The model under review builds one solid part; all positions refer to its coordinate system, in mm. Face numbers are marked on the shaded views. A direction names the side the tool comes from. Give positions to 0.01 mm unless a question says otherwise; leave off trailing zeros. Order: outer loops, then holes, each group sorted by start corner. A loop starts at its lowest first (then second) coordinate and runs counter-clockwise, first axis right, second up.
```python
from build123d import *

# Parameters (mm, degrees)
SKETCH1_W           = 16
SKETCH1_H           = 20
BOSS_EXTRUDE1_DEPTH = 15
SHELL1_T            = -2
SKETCH10_W          = 2
SKETCH10_H          = 16
BOSS_EXTRUDE4_DEPTH = 14
CUT_EXTRUDE2_REACH  = 32.726
SKETCH3_W           = 15
SKETCH3_H           = 6
CHAMFER1_SIZE       = 1
SKETCH4_W           = 4
SKETCH4_H           = 4
SKETCH4_W_2         = 22
SKETCH4_H_2         = 1.5
BOSS_EXTRUDE2_DEPTH = 2
CUT_EXTRUDE3_REACH  = 28.249
SKETCH5_W           = 12
SKETCH5_H           = 11.5
SKETCH8_R           = 1.75
CUT_EXTRUDE5_DEPTH  = 33.619012861
SKETCH9_R           = 3.25
CUT_EXTRUDE6_DEPTH  = 2.5


with BuildPart() as part:
    # Sketch1 → Boss-Extrude1 (new, symmetric)
    with BuildSketch(Plane.XY):
        Rectangle(SKETCH1_W, SKETCH1_H)
    extrude(amount=BOSS_EXTRUDE1_DEPTH, both=True)

    # Shell1
    shell1_openings = [part.faces().sort_by_distance(p)[0] for p in [
        (-8, 0, 0),
    ]]
    offset(amount=SHELL1_T, openings=shell1_openings, kind=Kind.INTERSECTION)

    # Sketch10 → Boss-Extrude4 (add)
    with BuildSketch(Plane.ZY.offset(-6)):
        with Locations((-12, 0)):
            Rectangle(SKETCH10_W, SKETCH10_H)
        with Locations((12, 0)):
            Rectangle(SKETCH10_W, SKETCH10_H)
    extrude(amount=BOSS_EXTRUDE4_DEPTH)

    # Sketch3 → Cut-Extrude2 (cut, up to next)
    with BuildSketch(Plane(origin=(8, 0, 9.25), x_dir=(0, 0, 1), z_dir=(-1, 0, 0)), mode=Mode.PRIVATE) as cut_extrude2_sk1:
        with Locations((-11.25, 1)):
            Rectangle(SKETCH3_W, SKETCH3_H)
    cut_extrude2_tool1 = extrude(cut_extrude2_sk1.sketch, amount=CUT_EXTRUDE2_REACH, mode=Mode.PRIVATE) & part.part
    add(cut_extrude2_tool1.solids().sort_by_distance((8, 1, -2))[0], mode=Mode.SUBTRACT)

    # Chamfer1
    chamfer1_edges = [part.edges().sort_by_distance(p)[0] for p in [
        (0, -10, 15),
        (8, 0, 15),
        (0, -10, -15),
        (0, 10, -15),
        (8, 0, -15),
        (0, 10, 15),
        (8, -10, 0),
        (8, 10, 0),
    ]]
    chamfer(chamfer1_edges, length=CHAMFER1_SIZE)

    # Sketch4 → Boss-Extrude2 (add)
    with BuildSketch(Plane.ZY.offset(-6)):
        with Locations((-9, 6)):
            Rectangle(SKETCH4_W, SKETCH4_H)
        with Locations((9, 6)):
            Rectangle(SKETCH4_W, SKETCH4_H)
        with Locations((0, -2.75)):
            Rectangle(SKETCH4_W_2, SKETCH4_H_2)
    extrude(amount=BOSS_EXTRUDE2_DEPTH)

    # Sketch5 → Cut-Extrude3 (cut, up to next)
    with BuildSketch(Plane.XZ.offset(10), mode=Mode.PRIVATE) as cut_extrude3_sk1:
        with Locations((-2, 5.25)):
            Rectangle(SKETCH5_W, SKETCH5_H)
    cut_extrude3_tool1 = extrude(cut_extrude3_sk1.sketch, amount=-CUT_EXTRUDE3_REACH, mode=Mode.PRIVATE) & part.part
    add(cut_extrude3_tool1.solids().sort_by_distance((-2, -10, 5.25))[0], mode=Mode.SUBTRACT)

    # Sketch8 → Cut-Extrude5 (cut, through all)
    with BuildSketch(Plane(origin=(0, 0, -15), x_dir=(-1, 0, 0), z_dir=(0, 0, -1))):
        with Locations((3.5, 0)):
            Circle(SKETCH8_R)
    extrude(amount=-CUT_EXTRUDE5_DEPTH, mode=Mode.SUBTRACT)

    # Sketch9 → Cut-Extrude6 (cut)
    with BuildSketch(Plane(origin=(0, 0, -15), x_dir=(-1, 0, 0), z_dir=(0, 0, -1))):
        with Locations((3.5, 0)):
            Circle(SKETCH9_R)
    cut_extrude6 = extrude(amount=-CUT_EXTRUDE6_DEPTH, mode=Mode.SUBTRACT)

    # Mirror1: Cut-Extrude6 across plane
    add(cut_extrude6.mirror(Plane.XY), mode=Mode.SUBTRACT)


solid = part.part
```
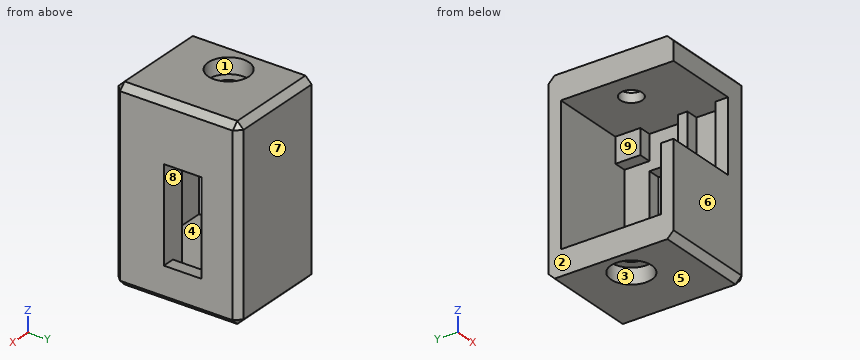
Item 1: Take a section at D-D (x = 0.75). Give the boundary of the cut face in (y, z).
Values found:
outline: (-10, -14) - (-9, -15) - (9, -15) - (10, -14) - (10, 14) - (9, 15) - (-9, 15) - (-10, 14) - (-10, 11) - (8, 11) - (8, -11) - (-8, -11) - (-8, -0.5) - (-10, -0.5) - close
Item 2: Clearance check with flat-ended pins moving along their axes: pin 1 Ø5 at (x, y) = (-3.5, 0) entering from +Z; pin 2 Ø5 at (x, y) = (-5, 0) entering from +Z; pin 3 Ø5 at (y, z) = (-5, 3.5) entering from -X; pin 4 Ø1 at (x, y) = (-4, -1.5) entering from -Z. State where each tip first meets the part, or that it passes through.
Values found:
pin 1: stops at z = 12.5
pin 2: stops at z = 15
pin 3: stops at x = 4
pin 4: stops at z = -12.5
Item 3: For the marked faces 1, 2, 3, 4 and 5, list the 3-axis set-ups (+Z, -Z, +X, -X, +Y, -Y) from which the entire face can be reached by the end or side of a thin tool; tool diameter is ignored.
Values found:
face 1: +Z
face 2: +Z, -Z, -X, +Y, -Y
face 3: -Z
face 4: -X
face 5: -Z, +X, -X, +Y, -Y
Item 4: Draft analysis for pull direction Y (two halves, no side actions). For the marked faces 6, 7, 8 and 9, state which applies: released by +Y, released by -Y, zero draft, split by the parting line, or undercut.
Values found:
face 6: released by -Y
face 7: released by +Y
face 8: undercut
face 9: zero draft
Item 5: For line 1 (Y direction, x = 5, z = -1); line 2 (Y direction, x = 2, z = -1.5); line 3 (Z direction, x = -5.25, y = -1), list the stretches that pass through material, from the lowest coordinate up.
Values found:
line 1: y = -10 to -8, -3.5 to -2, 8 to 10
line 2: y = -10 to -8, 8 to 10
line 3: z = -12.5 to -11, 11 to 12.5
Item 6: Take a section at A-A (y = 0). Give the number of separate pieces and of enclosed holes in the cut face, and give its area (3 significant figures).
Values found:
separate pieces: 4
enclosed holes: 0
area: 98.0 mm2
Item 7: Take a section at C-C (y = 2.5). Give the boundary of the cut face in (x, z).
Values found:
outline: (-8, -15) - (-5.58, -15) - (-5.58, -12.5) - (-1.42, -12.5) - (-1.42, -15) - (7, -15) - (8, -14) - (8, -9.5) - (6, -9.5) - (6, -11) - (-8, -11) - close; (-8, 11) - (6, 11) - (6, 5.5) - (8, 5.5) - (8, 14) - (7, 15) - (-1.42, 15) - (-1.42, 12.5) - (-5.58, 12.5) - (-5.58, 15) - (-8, 15) - close
